Could you check a few things on this drawing? It's one solid part, dimensions in mm from its lowest x, y, z. A direction names the side the tool comes from. Coordinates: 2 decimals unless noted, no trailing zeros. Order: outer loops, then holes, each group sorted by start corner. A loop starts at its lowest first (then second) coordinate and runs counter-clockwise, first axis right, second up. Notation, with made-up numbers: (39.5, 56.25) - (84.5, 56.25) arc R29 ccw to (84.5, 76.25) - close; hole circle Ø6 at (25, 87.25). An arc over 180 degrees is marked (long way). Answer in a Markdown table with one row per item. Add a question column.
Item 1: Will these pins go through, and if not, where does the flat tip stop? pin 1 Ø1.5 at (x, z) = (22, 8) entering from +Y; pin 2 Ø0.9 at (x, z) = (6, 5) entering from +Y.
Item 2: I want a section at D-D (z = 8). Please give me the cut outline in (x, y), plus the area to 3 significant figures.
Item 3: I want a section at B-B (x = 36.5). Please give me the cut outline in (y, z).
Item 4: On a 3-axis mill with a long thin cutter (end or side, diameter ignored), from which of +Z, -Z, +X, -X, +Y, -Y can I reach the whole of each face in a straight line? I mean the marked faces 1 and 2. Say none if no direction works.
Item 5: I want a section at A-A (z = 36.5). Please give me the cut outline in (x, y), plus the area to 3 significant figures.
Item 6: I want a section at C-C (z = 25). Please give me the cut outline in (x, y), plus the area to 3 significant figures.
Item 7: If I drill on line 1 along Z through (x, y) = (36.5, 36.85); line 2 along X through (y, z) = (38, 5), over which ranges is the centre line in solid material (lowest first)? Write a range as from..to.
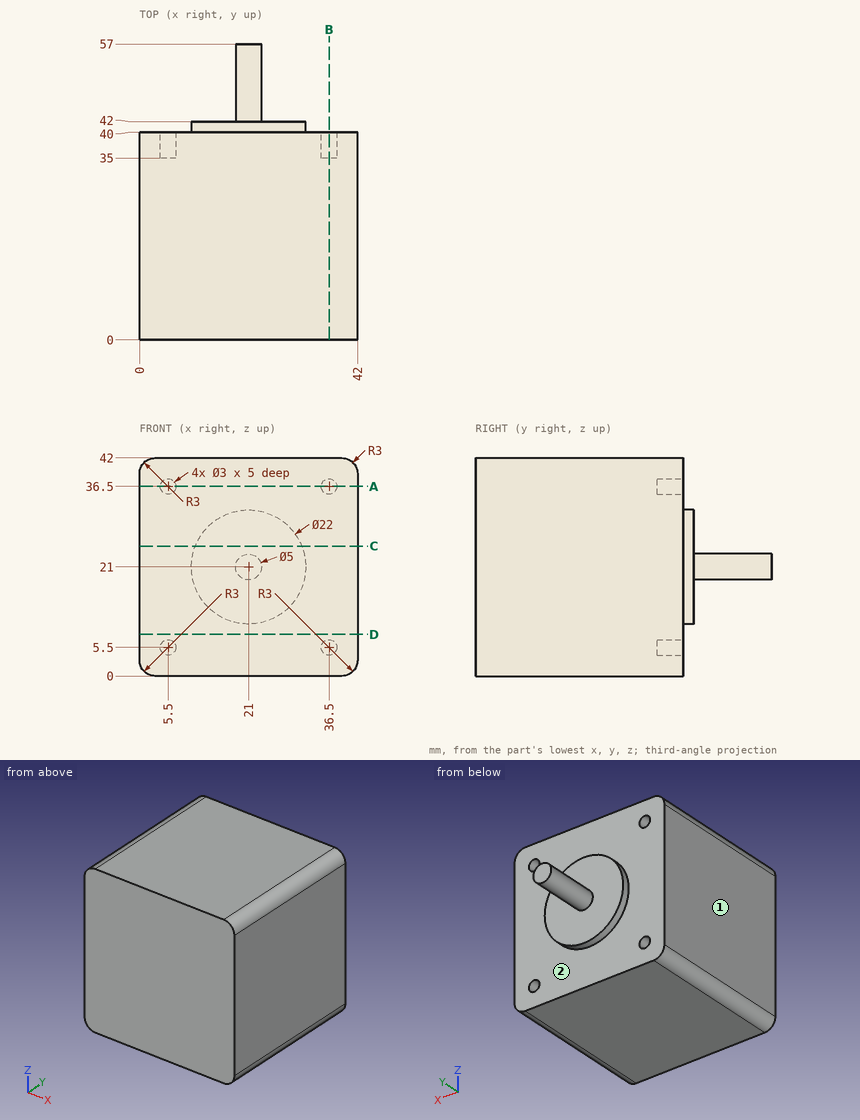
Values follow:
| question | item | result |
|---|---|---|
| 1 | pin 1 | stops at y = 40 |
| 1 | pin 2 | stops at y = 35 |
| 2 | outline | (0, 0) - (42, 0) - (42, 40) - (0, 40) - close |
| 2 | area | 1,680 mm^2 |
| 3 | outline | (0, 0) - (40, 0) - (40, 4) - (35, 4) - (35, 7) - (40, 7) - (40, 35) - (35, 35) - (35, 38) - (40, 38) - (40, 42) - (0, 42) - close |
| 4 | face 1 | +Z, -Z, -X, +Y, -Y |
| 4 | face 2 | +Y |
| 5 | outline | (0, 0) - (42, 0) - (42, 40) - (38, 40) - (38, 35) - (35, 35) - (35, 40) - (7, 40) - (7, 35) - (4, 35) - (4, 40) - (0, 40) - close |
| 5 | area | 1,650 mm^2 |
| 6 | outline | (0, 0) - (42, 0) - (42, 40) - (31.25, 40) - (31.25, 42) - (10.75, 42) - (10.75, 40) - (0, 40) - close |
| 6 | area | 1,720 mm^2 |
| 7 | line 1 | z = 0..4, 7..35, 38..42 |
| 7 | line 2 | x = 0..4.09, 6.91..35.09, 37.91..42 |
